Build history of the part. All positions in model axes, mm. Round coordinates to 2 decimals unless told otherwise and drop trailing zeros. Write each loop counter-clockwise with the first axis right and the second up, starting at its lowest first coordinate (ties: lowest second). Pieces come first, ordered by that corner, then holes.
1) Saw through at D-D (x = 88). Write the cut outline in (y, z), plus the area to 3 significant figures.
2) Wall check: probe 1 along X at (y, z) = (16, 11); probe 2 along X at (y, z) = (14, 10); probe 3 along Z at (x, y) = (156, -1). Give the ranges that are in metal, low to high.
3) Saw through at A-A (y = 14). Write the cut outline in (x, z), plus the area to 3 significant figures.
4) Saw through at B-B (y = 2). Write the cut outline in (x, z).
5) Pull direction X, two halves, no side cores. Call faces 1 (the flat face through (-58, 0, 10)), 2 (the flat face through (51, 30, 0)): +X half, -X half, draft (parallel to the pull), parting line (faces both ways), or undercut.
6) Saw through at C-C (x = 0). Write the cut outline in (y, z) (3 decimals), plus the area to 3 significant figures.
7) Flat gauge pins, fed straight in: pin 1 (12 mm diameter, centred on x = 40.5, y = 50.5, fed in from -Z); pin 2 (3 mm diameter, centred on y = 4, z = 14, fed in from +X); pin 3 (1.5 mm diameter, centred on x = 51.5, z = 2, fed in from +Y); pin 4 (5 mm diameter, centred on x = 128.5, z = 17.5, fed in from +Y). Where does each tip first touch, or does it go through?
from build123d import *

# Parameters (mm, degrees)
BOSS_EXTRUDE1_DEPTH = 20
SKETCH3_W           = 9
SKETCH3_H           = 14
BOSS_EXTRUDE2_DEPTH = 10
BOSS_EXTRUDE2_TAPER = 2


with BuildPart() as part:
    # Sketch2 → Boss-Extrude1 (new body)
    with BuildSketch(Plane.XY):
        with BuildLine():
            Line((45.085, 0), (60.085, 0))
            ThreePointArc((60.085, 0), (105.17, 45.085), (150.255, 0))
            Line((150.255, 0), (165.255, 0))
            ThreePointArc((165.255, 0), (120.18062124, 58.179794388), (52.585, 29.069313717))
            ThreePointArc((52.585, 29.069313717), (-15.01062124, 58.179794388), (-60.085, 0))
            Line((-60.085, 0), (-45.085, 0))
            ThreePointArc((-45.085, 0), (0, 45.085), (45.085, 0))
        make_face()
    extrude(amount=BOSS_EXTRUDE1_DEPTH)

    # Sketch3 → Boss-Extrude2 (add)
    with BuildSketch(Plane.XZ):
        with Locations((-52.585, 10)):
            Rectangle(SKETCH3_W, SKETCH3_H)
        with Locations((52.585, 10)):
            Rectangle(SKETCH3_W, SKETCH3_H)
        with Locations((157.755, 10)):
            Rectangle(SKETCH3_W, SKETCH3_H)
    extrude(amount=BOSS_EXTRUDE2_DEPTH, taper=BOSS_EXTRUDE2_TAPER)


solid = part.part
Evaluation:
1. outline: (41.69, 0) - (57.58, 0) - (57.58, 20) - (41.69, 20) - close
1. area: 318 mm2
2. probe 1: x = -57.92 to -42.15, 42.15 to 63.02, 147.32 to 163.09
2. probe 2: x = -58.43 to -42.86, 42.86 to 62.31, 148.03 to 163.6
2. probe 3: z = 3.03 to 16.97
3. outline: (-58.43, 0) - (-42.86, 0) - (-42.86, 20) - (-58.43, 20) - close; (42.86, 0) - (62.31, 0) - (62.31, 20) - (42.86, 20) - close; (148.03, 0) - (163.6, 0) - (163.6, 20) - (148.03, 20) - close
3. area: 1,010 mm2
4. outline: (-60.05, 0) - (-45.04, 0) - (-45.04, 20) - (-60.05, 20) - close; (45.04, 0) - (60.13, 0) - (60.13, 20) - (45.04, 20) - close; (150.21, 0) - (165.22, 0) - (165.22, 20) - (150.21, 20) - close
5. face 1: undercut
5. face 2: draft
6. outline: (45.085, 0) - (60.085, 0) - (60.085, 20) - (45.085, 20) - close
6. area: 300 mm2
7. pin 1: stops at z = 0
7. pin 2: stops at x = 165.2
7. pin 3: stops at y = 32.17
7. pin 4: stops at y = 56.36
